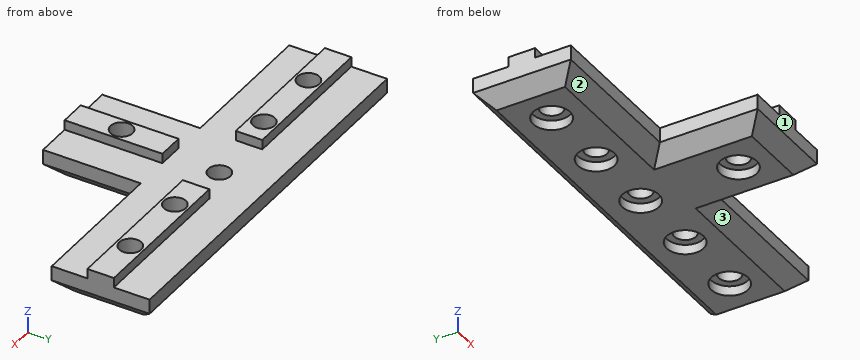
```python
from build123d import *

# Parameters (mm, degrees)
F1_DEPTH = 6
F2_W     = 30
F2_H     = 5.42
F3_DEPTH = 2
F4_R     = 2.25
F5_DEPTH = 8.001
F6_R     = 3.75
F7_DEPTH = 2
F8_SIZE  = 3


with BuildPart() as f1:
    # F0 (on Top) → F1 (new body)
    with BuildSketch(Plane.XY):
        Polygon((-40, 0), (-10, 0), (-10, -20), (0, -20), (10, -20), (10, 0), (40, 0), (40, 20), (0, 20), (-40, 20), align=None)
    extrude(amount=F1_DEPTH)

    # F2 (on face) → F3 (join)
    with BuildSketch(Plane.XY.offset(6)):
        Polygon((2.71, 0), (0, 0), (-2.71, 0), (-2.71, -20), (2.71, -20), align=None)
        Polygon((7.845558, 12.71), (7.845558, 10), (7.845558, 7.29), (40, 7.29), (40, 12.71), align=None)
        with Locations((-25, 10)):
            Rectangle(F2_W, F2_H)
    extrude(amount=F3_DEPTH)

    # F4 (on face) → F5 (cut, through all)
    with BuildSketch(Plane(origin=(0, 0, 0), x_dir=(1, 0, 0), z_dir=(0, 0, -1))):
        with Locations((-30, -10)):
            Circle(F4_R)
        with Locations((0, -10)):
            Circle(F4_R)
        with Locations((0, 10)):
            Circle(F4_R)
        with Locations((30, -10)):
            Circle(F4_R)
        with Locations((15, -10)):
            Circle(F4_R)
        with Locations((-15, -10)):
            Circle(F4_R)
    extrude(amount=-F5_DEPTH, mode=Mode.SUBTRACT)

    # F6 (on face) → F7 (cut)
    with BuildSketch(Plane(origin=(0, 0, 0), x_dir=(1, 0, 0), z_dir=(0, 0, -1))):
        with Locations((0, 10)):
            Circle(F6_R)
        with Locations((0, -10)):
            Circle(F6_R)
        with Locations((30, -10)):
            Circle(F6_R)
        with Locations((-30, -10)):
            Circle(F6_R)
        with Locations((-15, -10)):
            Circle(F6_R)
        with Locations((15, -10)):
            Circle(F6_R)
    extrude(amount=-F7_DEPTH, mode=Mode.SUBTRACT)

    # F8
    f8_edges = [f1.edges().sort_by_distance(p)[0] for p in [
        (-10, -10, 0),
        (-25, 0, 0),
        (10, -10, 0),
        (25, 0, 0),
        (0, 20, 0),
        (40, 10, 0),
        (-40, 10, 0),
        (0, -20, 0),
    ]]
    chamfer(f8_edges, length=F8_SIZE)


solid = f1.part
```
Geometry check sheet. Reference: the model listing, model coordinates, mm. Face numbers are marked on the shaded views. A direction names the side the tool comes from. Round coordinates to 2 decimals unless told otherwise and drop trailing zeros. Loops run counter-clockwise (first coordinate to the right, second up) from the corner with the lowest first, then second, coordinate; pieces in that order, holes last. Notation, with made-up numbers: (5.5, 29) - (31.5, 29) arc R27 ccw to (31.5, 67) - close; hole circle Ø1 at (-8.75, -29). An arc over 180 degrees is marked (long way). Write item = value, one per line. Start each with the question number.
1. Section check B-B on y = -10. Enter the section's corners in (x, z).
2. Set-up check for the marked faces 1, 2 and 3: record each of +Z, -Z, +X, -X, +Y, -Y from which the full face is reachable in a straight line by a thin tool's end or side.
3. Section check D-D on x = 15. Enter the section's corners in (y, z), then the cut area to 3 significant figures.
4. Depth check by flat-ended pin: pin 1 (1.6 mm diameter, centred on y = -13, z = 7, fed in from -X); pin 2 (2.5 mm diameter, centred on x = 32, z = 4, fed in from -Y); pin 3 (0.6 mm diameter, centred on x = 25, z = 7, fed in from +Y). Enter the tip coordinate at first touch or a pass-through.
5. Thickness scan on line 1 (X direction, y = 10, z = 3.35); line 2 (Y direction, x = 30, z = 3.2); line 3 (Y direction, x = 0, z = 2.25). Record the ranges inside material, lowest first.
6. Section check A-A on x = 0. Enter the section's corners in (y, z), then the cut area to 3 significant figures.
7. Section check C-C on z = 4.5. Enter the section's corners in (x, y).
Working result:
q1.outline = (-10, 3) - (-7, 0) - (-3.75, 0) - (-3.75, 2) - (-2.25, 2) - (-2.25, 8) - (-2.71, 8) - (-2.71, 6) - (-10, 6) - close; (2.25, 2) - (3.75, 2) - (3.75, 0) - (7, 0) - (10, 3) - (10, 6) - (2.71, 6) - (2.71, 8) - (2.25, 8) - close
q2.face_1 = +Z, -Z, +X, -X, -Y
q2.face_2 = -Z, -X, -Y
q2.face_3 = -Z, +X, -Y
q3.outline = (0, 3) - (3, 0) - (6.25, 0) - (6.25, 2) - (7.75, 2) - (7.75, 8) - (7.29, 8) - (7.29, 6) - (0, 6) - close; (12.25, 2) - (13.75, 2) - (13.75, 0) - (17, 0) - (20, 3) - (20, 6) - (12.71, 6) - (12.71, 8) - (12.25, 8) - close
q3.area = 79.8 mm^2
q4.pin_1 = -2.71
q4.pin_2 = 0
q4.pin_3 = 12.71
q5.line_1 = -40 to -32.25, -27.75 to -17.25, -12.75 to -2.25, 2.25 to 12.75, 17.25 to 27.75, 32.25 to 40
q5.line_2 = 0 to 7.75, 12.25 to 20
q5.line_3 = -19.25 to -12.25, -7.75 to 7.75, 12.25 to 19.25
q6.outline = (-20, 3) - (-17, 0) - (-13.75, 0) - (-13.75, 2) - (-12.25, 2) - (-12.25, 8) - (-20, 8) - close; (-7.75, 2) - (-6.25, 2) - (-6.25, 0) - (6.25, 0) - (6.25, 2) - (7.75, 2) - (7.75, 6) - (0, 6) - (0, 8) - (-7.75, 8) - close; (12.25, 2) - (13.75, 2) - (13.75, 0) - (17, 0) - (20, 3) - (20, 6) - (12.25, 6) - close
q6.area = 196 mm^2
q7.outline = (-40, 0) - (-10, 0) - (-10, -20) - (10, -20) - (10, 0) - (40, 0) - (40, 20) - (-40, 20) - close; hole circle Ø4.5 at (-30, 10); hole circle Ø4.5 at (-15, 10); hole circle Ø4.5 at (0, -10); hole circle Ø4.5 at (0, 10); hole circle Ø4.5 at (15, 10); hole circle Ø4.5 at (30, 10)
